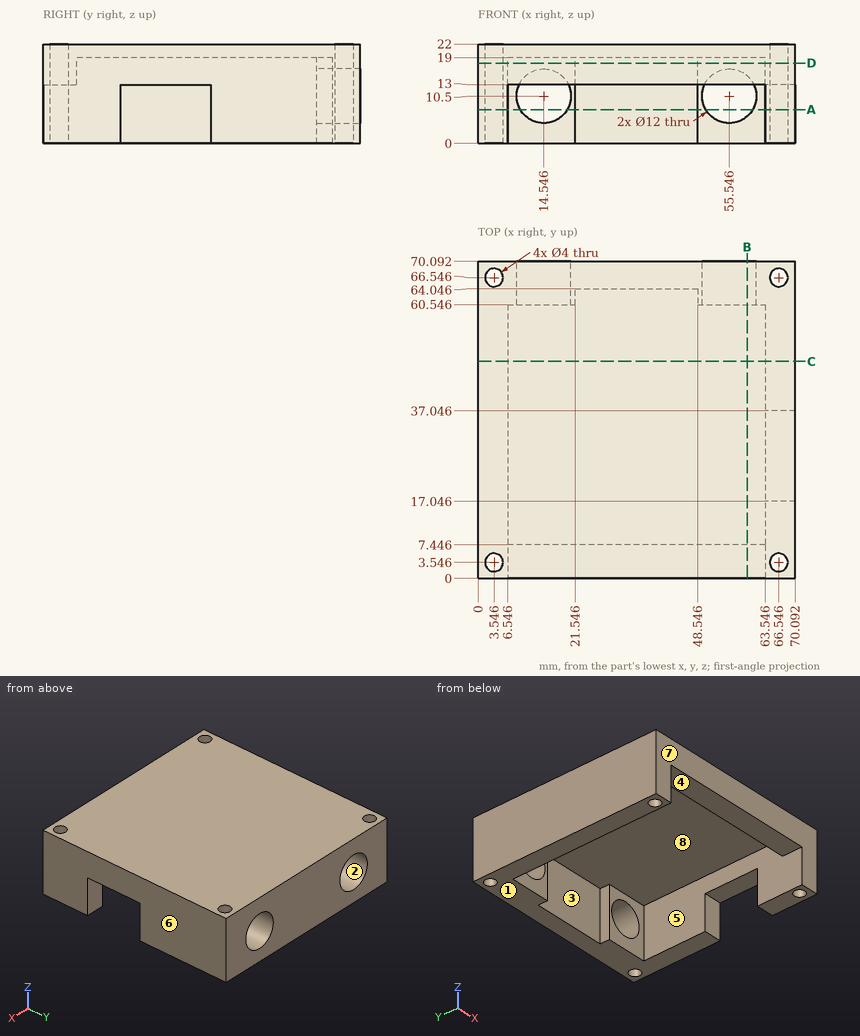
For this review, use the dimensioned drawing (mm, ordinates from the lowest corner) and the shaded views. A direction names the side the tool comes from. Round coordinates to 2 decimals unless told otherwise and drop trailing zeros. Order: outer loops, then holes, each group sorted by start corner. A loop starts at its lowest first (then second) coordinate and runs counter-clockwise, first axis right, second up. Notation, with made-up numbers: M -11.5,7 L 18.5,7 A21 cw 18.5,28 Z; hole C -37.5,-25.75 d4. An arc over 180 degrees is marked long. Use a Markdown table: item, result. Add a question column.
Item 1: Tool access review of the marked faces 1, 2, 3 and 4: name each direction out of +Z, -Z, +X, -X, +Y, -Y from which nothing blocks a thin tool from reaching the whole face with its end or side.
Item 2: Mouldability with a two-part tool opening along Y and no side actions: class the marked faces 5, 6, 7 and 8 as released by +Y, released by -Y, zero draft, split by the parting line, or undercut.
Item 3: Add section C-C, the plane y = 48. Give the boundary of the cut face in (x, z).
Item 4: Add section A-A, the plane z = 7.5. Give the boundary of the cut face in (x, y).
Item 5: To check wall thickness, follow line 1 along X through (y, z) = (64, 10.5); line 2 along X through (y, z) = (64.5, 10.5); line 3 along X through (y, z) = (54, 1.75). State the ranges of each line that lie inside material, in increasing order.
Item 6: Add section D-D, the plane z = 17.75. Give the boundary of the cut face in (x, y), then the cut area to 3 significant figures.
Item 7: Add section B-B, the plane x = 59.5. Give the boundary of the cut face in (y, z).
Item 8: Insertion check: pin 1 (2 mm diameter, centred on x = 13, y = 39.5, fed in from -Z); pin 2 (3.5 mm diameter, centred on x = 66.5, y = 29, fed in from -Z); pin 3 (12 mm diameter, centred on x = 55, z = 6, fed in from -Y). Each pin has a flat end and moves straight along its axis. Give the tip position at first contact, or say it passes through.
Geometry results:
| question | item | result |
|---|---|---|
| 1 | face 1 | -Z, +X, -X, +Y, -Y |
| 1 | face 2 | +Y |
| 1 | face 3 | -Z |
| 1 | face 4 | -Z, -Y |
| 2 | face 5 | undercut |
| 2 | face 6 | zero draft |
| 2 | face 7 | released by -Y |
| 2 | face 8 | undercut |
| 3 | outline | M 0,0 L 6.55,0 L 6.55,19 L 63.55,19 L 63.55,0 L 70.09,0 L 70.09,22 L 0,22 Z |
| 4 | outline | M 0,0 L 6.55,0 L 6.55,60.55 L 9.35,60.55 L 9.35,70.09 L 0,70.09 Z; M 19.74,60.55 L 21.55,60.55 L 21.55,64.05 L 48.55,64.05 L 48.55,60.55 L 50.35,60.55 L 50.35,70.09 L 19.74,70.09 Z; M 60.74,60.55 L 63.55,60.55 L 63.55,37.05 L 70.09,37.05 L 70.09,70.09 L 60.74,70.09 Z; M 63.55,0 L 70.09,0 L 70.09,17.05 L 63.55,17.05 Z; hole C 3.55,3.55 d4; hole C 3.55,66.55 d4; hole C 66.55,3.55 d4; hole C 66.55,66.55 d4 |
| 5 | line 1 | x = 0 to 8.55, 20.55 to 21.55, 48.55 to 49.55, 61.55 to 70.09 |
| 5 | line 2 | x = 0 to 8.55, 20.55 to 49.55, 61.55 to 70.09 |
| 5 | line 3 | x = 0 to 6.55, 63.55 to 70.09 |
| 6 | outline | M 0,0 L 70.09,0 L 70.09,70.09 L 0,70.09 Z; hole C 3.55,3.55 d4; hole C 3.55,66.55 d4; hole M 6.55,7.45 L 63.55,7.45 L 63.55,60.55 L 48.55,60.55 L 48.55,64.05 L 21.55,64.05 L 21.55,60.55 L 6.55,60.55 Z; hole C 66.55,3.55 d4; hole C 66.55,66.55 d4 |
| 6 | area | 1,740 mm² |
| 7 | outline | M 0,13 L 7.45,13 L 7.45,19 L 60.55,19 L 60.55,15.01 L 70.09,15.01 L 70.09,22 L 0,22 Z; M 60.55,0 L 70.09,0 L 70.09,5.99 L 60.55,5.99 Z |
| 8 | pin 1 | stops at z = 19 |
| 8 | pin 2 | stops at z = 13 |
| 8 | pin 3 | stops at y = 60.55 |
